Model file for the job. Use its own axes, mm. A direction names the side the tool comes from. Coordinates: 2 decimals unless noted, no trailing zeros. Write each loop counter-clockwise with the first axis right and the second up, starting at its lowest first coordinate (ties: lowest second). Pieces come first, ordered by that corner, then holes. Notation, with made-up numbers: (-12.5, 43.5) - (8.5, 43.5) arc R22 ccw to (8.5, 60.5) - close; hole circle Ø1 at (61, 17.5). An arc over 180 degrees is marked (long way). Put each result on its own line as item: value. Start each with the question number.
1. Saw through at C-C, the plane z = -10. Write the cut outline in (x, y), plus the area to 3 significant figures.
2. Saw through at B-B, the plane x = -2.5. Write the cut outline in (y, z).
3. Drill centre lines: L1, parallel to Y at x = -5.5, z = -27.7; L2, parallel to Y at x = -5.5, z = -28.55; L3, parallel to X at y = 25.5, z = -9. Where is each one in solid material? Low to high. Write a range as from..to.
4. Drop flat-ended pins along their axis: P1, Ø18, axis at y = 17, z = -8.5, coming from the -X side; P2, Ø2, axis at x = -4.5, y = 24.5, coming from the +Z side; P3, Ø1.2, axis at y = 33, z = 1.5, coming from the +X side. Give the stop position or say it passes through.
5. Pull direction Y, two halves, no side cores. Call faces 4 (the face through (0, 18, -8)), 5 (the face through (4.01, 34.24, 1.16)), 6 (the face through (-5.164, 32.487, -28.028)), 7 (the face through (-8, 36, -29)): released by +Y, released by -Y, zero draft, split by the parting line, or undercut.
6. Saw through at D-D, the plane y = 18.5. Write the cut outline in (x, z), plus the area to 3 significant figures.
7. Saw through at A-A, the plane y = 3. Write the cut outline in (x, z).
8. Which spindle directions (+Z, -Z, +X, -X, +Y, -Y) get a long thin tool onto all of the face, cutting with end or side? Do faces 1 (the face through (-8, 18, -26)), 2 (the face through (4, 18, -21.84)), 3 (the face through (4.5, 18, -1)). Say none if no direction does.
```python
from build123d import *

# Parameters (mm, degrees)
SKETCH1_W           = 30
SKETCH1_H           = 37
BOSS_EXTRUDE1_DEPTH = 4.5
SKETCH2_W           = 4
SKETCH2_H           = 37
BOSS_EXTRUDE2_DEPTH = 42
SKETCH3_W           = 30
SKETCH3_H           = 37
BOSS_EXTRUDE3_DEPTH = 4.5
SKETCH8_R           = 11.1
CUT_EXTRUDE1_DEPTH  = 4
SKETCH9_R           = 1.55
CUT_EXTRUDE2_DEPTH  = 4
CHAMFER3_SIZE       = 2
SKETCH_6_R          = 7.5
EXTRUDE_2_DEPTH     = 5.5
SKETCH_5_R          = 4
EXTRUDE_1_DEPTH     = 20.5
SKETCH_15_R         = 8.5
EXTRUDE_6_DEPTH     = 0.5
EXTRUDE_START       = 0.5
SKETCH_16_R         = 8.5
SKETCH_16_R_2       = 7.45
EXTRUDE_7_DEPTH     = 0.5
SKETCH_17_W         = 4.5
SKETCH_17_H         = 37
EXTRUDE_8_DEPTH     = 10
SKETCH_23_R         = 1.25
CUT_EXTRUDE_4_DEPTH = 1
EXTRUDE_START_2     = -20.5
EXTRUDE_11_DEPTH    = 20.5
CUT_EXTRUDE_5_DEPTH = 67.219332525
SKETCH_27_W         = 8.159891724
SKETCH_27_H         = 2
CUT_EXTRUDE_6_DEPTH = 2


with BuildPart() as part:
    # Sketch1 → Boss-Extrude1 (new body)
    with BuildSketch(Plane(origin=(0, 0, 0), x_dir=(0, 0, -1), z_dir=(1, 0, 0))):
        with Locations((15, 18.5)):
            Rectangle(SKETCH1_W, SKETCH1_H)
    extrude(amount=BOSS_EXTRUDE1_DEPTH)

    # Sketch2 → Boss-Extrude2 (add)
    with BuildSketch(Plane.ZY):
        with Locations((-28, 18.5)):
            Rectangle(SKETCH2_W, SKETCH2_H)
    extrude(amount=BOSS_EXTRUDE2_DEPTH)

    # Sketch3 → Boss-Extrude3 (add)
    with BuildSketch(Plane.ZY.offset(42)):
        with Locations((-15, 18.5)):
            Rectangle(SKETCH3_W, SKETCH3_H)
    extrude(amount=BOSS_EXTRUDE3_DEPTH)

    # Sketch8 → Cut-Extrude1 (cut)
    with BuildSketch(Plane.XY.offset(-26)):
        with Locations((-21, 18.5)):
            Circle(SKETCH8_R)
    extrude(amount=-CUT_EXTRUDE1_DEPTH, mode=Mode.SUBTRACT)

    # Sketch9 → Cut-Extrude2 (cut)
    with BuildSketch(Plane(origin=(0, 0, -30), x_dir=(-1, 0, 0), z_dir=(0, 0, -1))):
        with Locations((5.5, 34)):
            Circle(SKETCH9_R)
        with Locations((36.5, 34)):
            Circle(SKETCH9_R)
        with Locations((36.5, 3)):
            Circle(SKETCH9_R)
        with Locations((5.5, 3)):
            Circle(SKETCH9_R)
    extrude(amount=-CUT_EXTRUDE2_DEPTH, mode=Mode.SUBTRACT)

    # Chamfer3
    # the kernel refuses this chamfer: 2 mm, written as the material it takes off along each edge
    with BuildSketch(Plane(origin=(4.5, -5.143365976, -30), x_dir=(0.02749587661058651, 0, 0.9996219169112968), z_dir=(0, 1, 0))) as chamfer3_piece_1:
        Polygon((CHAMFER3_SIZE * 0.999621916911, -CHAMFER3_SIZE * 0.0274958766106), (-CHAMFER3_SIZE * 0.0274958766106, -CHAMFER3_SIZE * 0.999621916911), (0, 0), align=None)
    extrude(amount=47.286731952, mode=Mode.SUBTRACT)
    with BuildSketch(Plane(origin=(-46.5, 42.143365976, -30), x_dir=(0.9996219169112968, 0, -0.027495876610585647), z_dir=(0, -1, 0))) as chamfer3_piece_2:
        Polygon((CHAMFER3_SIZE * 0.999621916911, CHAMFER3_SIZE * 0.0274958766106), (-CHAMFER3_SIZE * 0.0274958766106, CHAMFER3_SIZE * 0.999621916911), (0, 0), align=None)
    extrude(amount=47.286731952, mode=Mode.SUBTRACT)
    with BuildSketch(Plane(origin=(-51.643365976, 37, -30), x_dir=(0, -0.9996219169112968, -0.027495876610585647), z_dir=(1, 0, 0)), Plane(origin=(-51.643365976, 0, -30), x_dir=(0, -0.02749587661058639, 0.9996219169112968), z_dir=(1, 0, 0))) as chamfer3_piece_3:
        Polygon((CHAMFER3_SIZE * 0.999621916911, -CHAMFER3_SIZE * 0.0274958766106), (-CHAMFER3_SIZE * 0.0274958766106, -CHAMFER3_SIZE * 0.999621916911), (0, 0), align=None)
    extrude(amount=61.286731952, mode=Mode.SUBTRACT)

    # 草图6 → 凸台-拉伸2 (add)
    with BuildSketch(Plane(origin=(4.5, 0, 0), x_dir=(0, 0, -1), z_dir=(1, 0, 0))):
        with Locations((10, 18.5)):
            Circle(SKETCH_6_R)
    extrude(amount=EXTRUDE_2_DEPTH)

    # 草图5 → 凸台-拉伸1 (add)
    with BuildSketch(Plane.ZY.offset(46.5)):
        with Locations((-10, 18.5)):
            Circle(SKETCH_5_R)
    extrude(amount=EXTRUDE_1_DEPTH)

    # 草图15 → 凸台-拉伸6 (add)
    with BuildSketch(Plane.ZY.offset(46.5)):
        with Locations((-10, 18.5)):
            Circle(SKETCH_15_R)
    extrude(amount=EXTRUDE_6_DEPTH)

    # 草图16 → 凸台-拉伸7 (add)
    with BuildSketch(Plane(origin=(4.5, 0, 0), x_dir=(0, 0, -1), z_dir=(1, 0, 0)).offset(EXTRUDE_START)):
        with Locations(Location((10, 18.5, 0), (0, 0, 180))):
            Circle(SKETCH_16_R)
        with Locations((10, 18.5)):
            Circle(SKETCH_16_R_2, mode=Mode.SUBTRACT)
    extrude(amount=-EXTRUDE_7_DEPTH)

    # 草图17 → 凸台-拉伸8 (add)
    with BuildSketch(Plane.XY):
        with Locations((2.25, 18.5)):
            Rectangle(SKETCH_17_W, SKETCH_17_H)
    extrude(amount=EXTRUDE_8_DEPTH)

    # 草图23 → 切除-拉伸4 (cut)
    with BuildSketch(Plane(origin=(4.5, 0, 0), x_dir=(0, 0, -1), z_dir=(1, 0, 0))):
        with Locations((-1, 33)):
            Circle(SKETCH_23_R)
    extrude(amount=-CUT_EXTRUDE_4_DEPTH, mode=Mode.SUBTRACT)

    # 草图26 → 凸台-拉伸11 (add)
    with BuildSketch(Plane.ZY.offset(67).offset(EXTRUDE_START_2)):
        with BuildLine():
            ThreePointArc((-8.063508327, 22), (-10, 23.5), (-11.936491673, 22))
            ThreePointArc((-11.936491673, 22), (-10, 22.5), (-8.063508327, 22))
        make_face()
        with BuildLine():
            ThreePointArc((-13.5, 16.563508327), (-14, 18.5), (-13.5, 20.436491673))
            ThreePointArc((-13.5, 20.436491673), (-15, 18.5), (-13.5, 16.563508327))
        make_face()
        with BuildLine():
            ThreePointArc((-6.5, 16.563508327), (-5, 18.5), (-6.5, 20.436491673))
            ThreePointArc((-6.5, 20.436491673), (-6, 18.5), (-6.5, 16.563508327))
        make_face()
        with BuildLine():
            ThreePointArc((-8.063508327, 15), (-10, 14.5), (-11.936491673, 15))
            ThreePointArc((-11.936491673, 15), (-10, 13.5), (-8.063508327, 15))
        make_face()
    extrude(amount=EXTRUDE_11_DEPTH)

    # 草图25 → 切除-拉伸5 (cut, through all)
    with BuildSketch(Plane.ZY.offset(21)):
        Polygon((21.58280616, 37.67604856), (19.928852176, -12.32395144), (-38.530236753, -10.39017858), (-38.530236753, 37.67604856), align=None)
    extrude(amount=CUT_EXTRUDE_5_DEPTH, mode=Mode.SUBTRACT)

    # 草图27 → 切除-拉伸6 (cut)
    with BuildSketch(Plane(origin=(4.5, 0, 0), x_dir=(0, 0, -1), z_dir=(1, 0, 0))):
        with Locations((25.920054138, 18.5)):
            Rectangle(SKETCH_27_W, SKETCH_27_H)
    extrude(amount=-CUT_EXTRUDE_6_DEPTH, mode=Mode.SUBTRACT)


solid = part.part
```
Final values:
1. outline: (0, 0) - (4.5, 0) - (4.5, 10) - (5, 10) - (5, 11) - (10, 11) - (10, 26) - (5, 26) - (5, 27) - (4.5, 27) - (4.5, 37) - (0, 37) - close
1. area: 250 mm²
2. outline: (0, -28) - (2, -30) - (35, -30) - (37, -28) - (37, -26) - (0, -26) - close
3. L1: y = 0..1.45, 4.55..32.45, 35.55..37
3. L2: y = 0.55..1.45, 4.55..32.45, 35.55..36.45
3. L3: x = 0..10
4. P1: stops at x = 0
4. P2: stops at z = -26
4. P3: stops at x = 3.5
5. face 4: zero draft
5. face 5: undercut
5. face 6: undercut
5. face 7: released by +Y
6. outline: (-9.9, -30) - (2.5, -30) - (2.5, -21.84) - (4.5, -21.84) - (4.5, -18.5) - (5, -18.5) - (5, -17.5) - (10, -17.5) - (10, -2.5) - (5, -2.5) - (5, -1.5) - (4.5, -1.5) - (4.5, 10) - (0, 10) - (0, -26) - (-9.9, -26) - close
6. area: 287 mm²
7. outline: (-21, -30) - (-7.05, -30) - (-7.05, -26) - (-21, -26) - close; (-3.95, -30) - (2.5, -30) - (4.5, -28) - (4.5, 10) - (0, 10) - (0, -26) - (-3.95, -26) - close
8. face 1: +Z, -X, +Y, -Y
8. face 2: -Z, +X
8. face 3: +X
